CAD build for the part. Positions are in the model's coordinates, mm. A direction names the side the tool comes from. Round coordinates to 2 decimals unless told otherwise and drop trailing zeros. Loops run counter-clockwise (first coordinate to the right, second up) from the corner with the lowest first, then second, coordinate; pieces in that order, holes last. Notation, with made-up numbers: (13, -18) - (42, -18) arc R23 ccw to (42, -10) - close; hole circle Ø7 at (50.25, 22). An arc over 180 degrees is marked (long way). Use one line per item in the form item = value.
from build123d import *

# Parameters (mm, degrees)
SKETCH1_R           = 20
BOSS_EXTRUDE1_DEPTH = 150
SKETCH2_R           = 4
BOSS_EXTRUDE2_DEPTH = 30


with BuildPart() as part:
    # Sketch1 → Boss-Extrude1 (new body)
    with BuildSketch(Plane(origin=(0, 0, 0), x_dir=(1, 0, 0), z_dir=(0, 1, 0))):
        with Locations(Location((0, 0, 0), (0, 0, 270))):
            Circle(SKETCH1_R)
    extrude(amount=BOSS_EXTRUDE1_DEPTH)

    # Sketch2 → Boss-Extrude2 (add)
    with BuildSketch(Plane.XZ):
        with Locations(Location((0, 0, 0), (0, 0, 90))):
            Circle(SKETCH2_R)
    boss_extrude2 = extrude(amount=BOSS_EXTRUDE2_DEPTH)

    # Mirror1: Boss-Extrude2 across plane
    add(boss_extrude2.mirror(Plane(origin=(0, 75, 0), x_dir=(0, 0, 1), z_dir=(0, -1, 0))))


solid = part.part
1) Slice it at C-C (y = 24.5). Write the cut outline in (x, z).
Report:
outline = circle Ø40 at (0, 0)
2) Slice it at B-B (z = 0). Write the cut outline in (x, y).
Report:
outline = (-20, 0) - (-4, 0) - (-4, -30) - (4, -30) - (4, 0) - (20, 0) - (20, 150) - (4, 150) - (4, 180) - (-4, 180) - (-4, 150) - (-20, 150) - close
3) Slice it at D-D (x = 15). Write the cut outline in (y, z).
Report:
outline = (0, -13.23) - (150, -13.23) - (150, 13.23) - (0, 13.23) - close
4) Drill centre lines: probe 1 along Y at (x, z) = (-12.5, -14.5); probe 2 along X at (y, z) = (102.5, -1); probe 3 along X at (y, z) = (40, -9.5). Where is each one in solid material? Low to high.
Report:
probe_1 = 0 to 150
probe_2 = -19.97 to 19.97
probe_3 = -17.6 to 17.6
5) Tool access for faces 1 (the cylindrical face through (3.905, -14.79, -0.867)), 2 (the cylindrical face through (3.905, 164.79, -0.867)), 3 (the cylindrical face through (-19.524, 73.95, -4.336)): list every direction of +Z, -Z, +X, -X, +Y, -Y with a clear straight run to the whole face (end or side of a thin tool).
Report:
face_1 = -Y
face_2 = +Y
face_3 = +Y, -Y
6) Slice it at A-A (x = 0). Write the cut outline in (y, z).
Report:
outline = (-30, -4) - (0, -4) - (0, -20) - (150, -20) - (150, -4) - (180, -4) - (180, 4) - (150, 4) - (150, 20) - (0, 20) - (0, 4) - (-30, 4) - close
7) Flat gauge pins, fed straight in: pin 1 (4 mm diameter, centred on x = -15, y = 86, fed in from +Z); pin 2 (5 mm diameter, centred on y = 12, z = 7, fed in from +X); pin 3 (3 mm diameter, centred on x = 14, y = 127, fed in from -Z). Where does each tip first touch, or does it go through?
Report:
pin_1 = 15.2
pin_2 = 19.49
pin_3 = -15.61
